Could you check a few things on this model? Use its own coordinates, in mm. Face numbers are marked on the shaded views. Coordinates: 2 decimals unless noted, no trailing zeros. Order: outer loops, then holes, each group sorted by start corner. A loop starts at its lowest first (then second) coordinate and runs counter-clockwise, first axis right, second up. Notation, with made-up numbers: (-27.75, 61.5) - (-11.75, 61.5) arc R25 cw to (-11.75, 83.5) - close; hole circle Ø1 at (31.25, 53). An arc over 180 degrees is marked (long way). Answer as CSV lines item,"result". Start each with the question number.
1. I want a section at A-A, the plane x = 0. List the corners of the cut face in (y, z) for me.
2. Thinking about a two-plate mould opening in Z: for the marked faces 1 and 2, which applies, released by +Z, released by -Z, zero draft, split by the parting line, or undercut?
3. For pin 1 (4 mm diameter, centred on y = 15.5, z = -13.5, fed in from -X); pin 2 (4 mm diameter, centred on y = 6, z = -16.5, fed in from -X); pin 3 (3 mm diameter, centred on y = 12, z = 27.5, fed in from -X), each with a flat end and sliding along its axis, tell me the tip position at first contact or that it passes through.
4. I want a section at B-B, the plane z = 0. List the corners of the cut face in (x, y) for me.
5. I need wall thicknesses on probe 1 along X at (y, z) = (9.5, 0); probe 2 along X at (y, z) = (6.5, -21.5); probe 3 along Z at (x, y) = (-22.5, 6.5). Which ranges of each line are inside material? Lowest first, please.
6. I want a section at C-C, the plane y = 8. List the corners of the cut face in (x, z) for me, and give its area (3 significant figures).
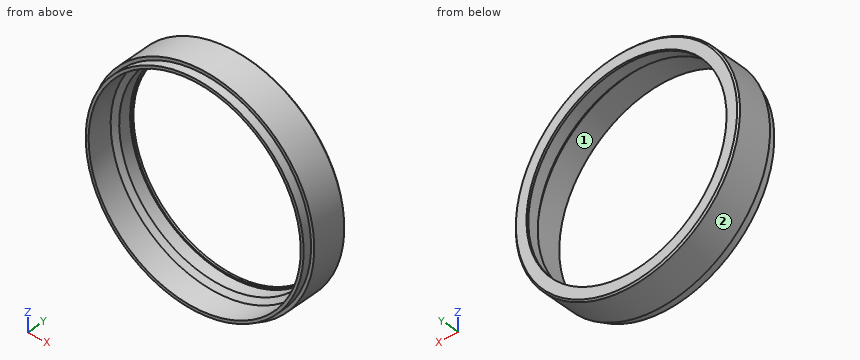
from build123d import *


with BuildPart() as part:
    # Sketch1 → Revolve1 (revolve)
    with BuildSketch(Plane.XY, mode=Mode.PRIVATE) as revolve1_sk:
        Polygon((-35, 3.2), (-35, 11.5), (-33.5, 13), (-33.5, 17.1), (-33, 17.1), (-33, 17.8), (-36.5, 17.8), (-37, 17.3), (-37, 6), (-35.95, 6), (-35.95, 3.2), align=None)
    revolve(revolve1_sk.sketch.rotate(Axis((0, 0, 0), (0, -1, 0)), 270), axis=Axis((0, 0, 0), (0, -1, 0)))


solid = part.part
Solved:
1,outline,"(3.2, -35.95) - (6, -35.95) - (6, -37) - (17.3, -37) - (17.8, -36.5) - (17.8, -33) - (17.1, -33) - (17.1, -33.5) - (13, -33.5) - (11.5, -35) - (3.2, -35) - close; (3.2, 35) - (11.5, 35) - (13, 33.5) - (17.1, 33.5) - (17.1, 33) - (17.8, 33) - (17.8, 36.5) - (17.3, 37) - (6, 37) - (6, 35.95) - (3.2, 35.95) - close"
2,face 1,"undercut"
2,face 2,"split by the parting line"
3,pin 1,"stops at x = -35.17"
3,pin 2,"stops at x = -34.04"
3,pin 3,"stops at x = -26.32"
4,outline,"(-37, 6) - (-35.95, 6) - (-35.95, 3.2) - (-35, 3.2) - (-35, 11.5) - (-33.5, 13) - (-33.5, 17.1) - (-33, 17.1) - (-33, 17.8) - (-36.5, 17.8) - (-37, 17.3) - close; (33, 17.1) - (33.5, 17.1) - (33.5, 13) - (35, 11.5) - (35, 3.2) - (35.95, 3.2) - (35.95, 6) - (37, 6) - (37, 17.3) - (36.5, 17.8) - (33, 17.8) - close"
5,probe 1,"x = -37 to -35, 35 to 37"
5,probe 2,"x = -30.11 to -27.62, 27.62 to 30.11"
5,probe 3,"z = -29.37 to -26.81, 26.81 to 29.37"
6,outline,"circle Ø74 at (0, 0); hole circle Ø70 at (0, 0)"
6,area,"452 mm2"
